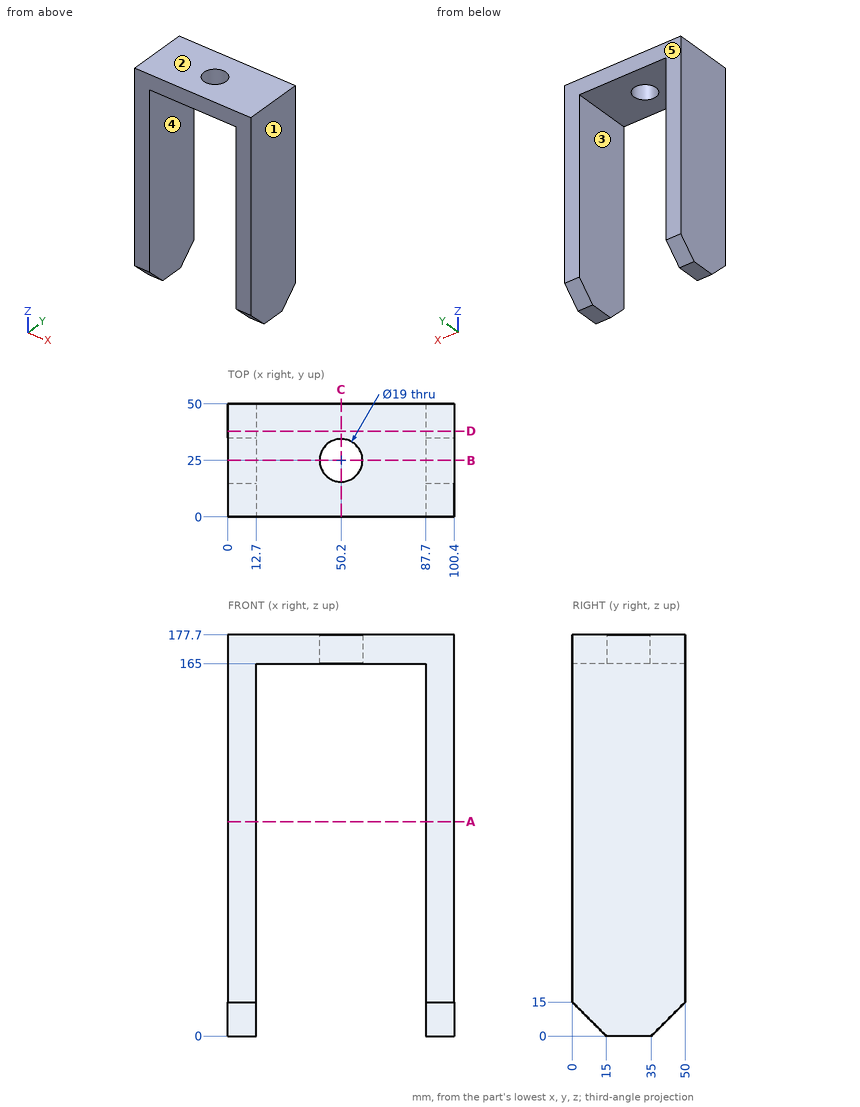
The drawing under review shows one solid part. Ordinate dimensions are in mm from its lowest x, y, z. A direction names the side the tool comes from. Coordinates: 2 decimals unless noted, no trailing zeros. Order: outer loops, then holes, each group sorted by start corner. A loop starts at its lowest first (then second) coordinate and runs counter-clockwise, first axis right, second up. Notation, with made-up numbers: (-11, 66) -> (33, 66) arc R28 cw to (33, 98) -> close; hole circle Ø3 at (24, 74.25). An arc over 180 degrees is marked (long way). Answer in a Markdown table with one row per item. Add a question column.
Item 1: Machinability: for the marked faces 4 and 5, which of the approach directions +Z, -Z, +X, -X, +Y, -Y give a long, thin tool a straight path to every point of the face, cutting with its end or side? Answer none if there is none.
Item 2: To check wall thickness, follow probe 1 along Y at (x, z) = (50.2, 173.25); probe 2 along X at (y, z) = (47, 110); probe 3 along Z at (x, y) = (78, 4.5). State the ranges of each line that lie inside material, in increasing order.
Item 3: We need section B-B on y = 25. Write out the cut boundary in (x, z), plus the area to 3 significant figures.
Item 4: We need section D-D on y = 38. Write out the cut boundary in (x, z).
Item 5: We need section C-C on x = 50.2. Write out the cut boundary in (y, z), plus the area to 3 significant figures.
Item 6: Mouldability with a two-part tool opening along X and no side actions: class the marked faces 1, 2 and 3 as +X half, -X half, draft (parallel to the pull), parting line (faces both ways), or undercut.
Item 7: We need section A-A on z = 95. Write out the cut boundary in (x, y).
Item 8: Clearance check with flat-ended pins moving along their axes: pin 1 (25 mm diameter, centred on x = 59, y = 36.5, fed in from -Z); pin 2 (15 mm diameter, centred on x = 50.2, y = 25, fed in from -Z). State where each tip first meets the part, or that it passes through.
Final values:
| question | item | result |
|---|---|---|
| 1 | face 4 | -Z, +Y, -Y |
| 1 | face 5 | +Z, -Z, +X, -X, +Y |
| 2 | probe 1 | y = 0 to 15.5, 34.5 to 50 |
| 2 | probe 2 | x = 0 to 12.7, 87.7 to 100.4 |
| 2 | probe 3 | z = 165 to 177.7 |
| 3 | outline | (0, 0) -> (12.7, 0) -> (12.7, 165) -> (40.7, 165) -> (40.7, 177.7) -> (0, 177.7) -> close; (59.7, 165) -> (87.7, 165) -> (87.7, 0) -> (100.4, 0) -> (100.4, 177.7) -> (59.7, 177.7) -> close |
| 3 | area | 5,220 mm2 |
| 4 | outline | (0, 3) -> (12.7, 3) -> (12.7, 165) -> (87.7, 165) -> (87.7, 3) -> (100.4, 3) -> (100.4, 177.7) -> (0, 177.7) -> close |
| 5 | outline | (0, 165) -> (15.5, 165) -> (15.5, 177.7) -> (0, 177.7) -> close; (34.5, 165) -> (50, 165) -> (50, 177.7) -> (34.5, 177.7) -> close |
| 5 | area | 394 mm2 |
| 6 | face 1 | +X half |
| 6 | face 2 | draft |
| 6 | face 3 | undercut |
| 7 | outline | (0, 0) -> (12.7, 0) -> (12.7, 50) -> (0, 50) -> close; (87.7, 0) -> (100.4, 0) -> (100.4, 50) -> (87.7, 50) -> close |
| 8 | pin 1 | stops at z = 165 |
| 8 | pin 2 | passes through |
